Can you work these out from the drawing? Everything is in mm from the part's minimum corner. A direction names the side the tool comes from. Coordinates: 2 decimals unless noted, no trailing zeros. Order: outer loops, then holes, each group sorted by start corner. A loop starts at its lowest first (then second) coordinate and runs counter-clockwise, first axis right, second up. Notation, with made-up numbers: (9, 0.5) - (54, 0.5) arc R20 ccw to (54, 25.5) - close; hole circle Ø3 at (81, 55). An arc over 180 degrees is marked (long way). One line per item, written item: value.
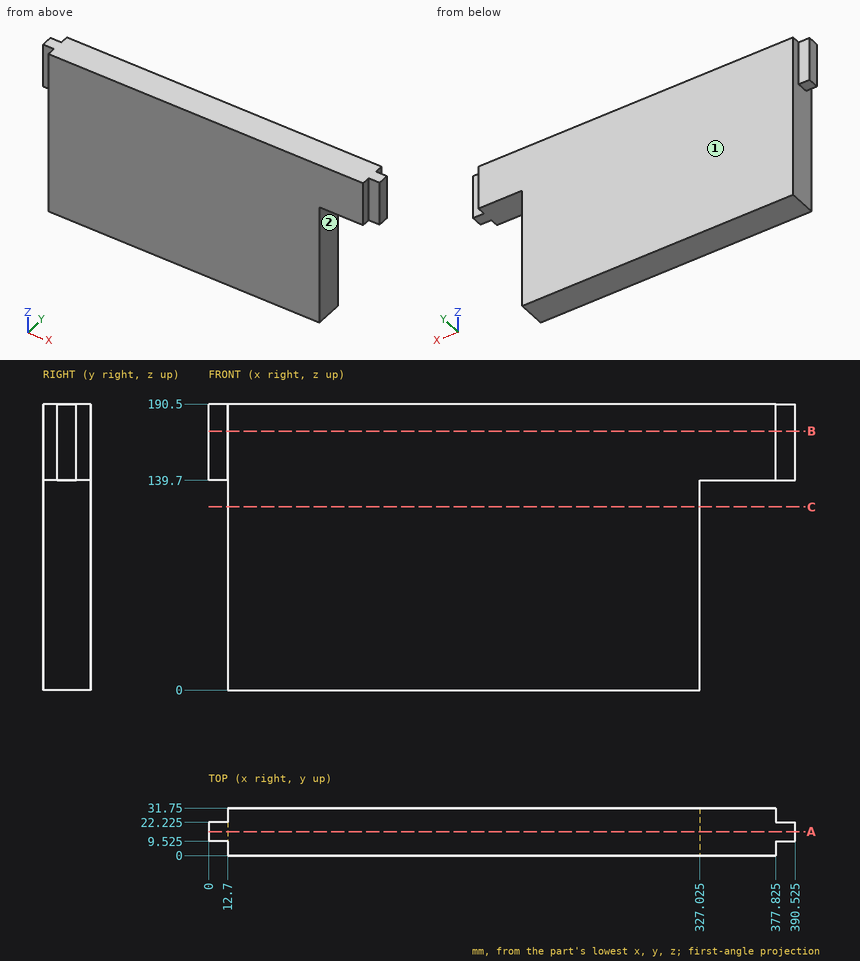
Item 1: I want a section at B-B on z = 172.5. Please give me the cut outline in (x, y) (3 decimals).
Conclusion:
outline: (0, 9.525) - (12.7, 9.525) - (12.7, 0) - (377.825, 0) - (377.825, 9.525) - (390.525, 9.525) - (390.525, 22.225) - (377.825, 22.225) - (377.825, 31.75) - (12.7, 31.75) - (12.7, 22.225) - (0, 22.225) - close
Item 2: I want a section at C-C on z = 122. Please give me the cut outline in (x, y) (3 decimals).
Conclusion:
outline: (12.7, 0) - (327.025, 0) - (327.025, 31.75) - (12.7, 31.75) - close
Item 3: I want a section at A-A on y = 16. Please give me the cut outline in (x, z) (3 decimals).
Conclusion:
outline: (0, 139.7) - (12.7, 139.7) - (12.7, 0) - (327.025, 0) - (327.025, 139.7) - (390.525, 139.7) - (390.525, 190.5) - (0, 190.5) - close
Item 4: For the marked faces 1 and 2, which set-ups out of +Z, -Z, +X, -X, +Y, -Y let a thin tool reach every point of the face, with its end or its side?
Conclusion:
face 1: +Z, -Z, +X, -X, +Y
face 2: -Z, +X, +Y, -Y
Item 5: I'm going to push flat-ended pins straight in: pin 1 Ø6.5 at (x, z) = (7.5, 177.5) entering from +Y (3 decimals); pin 2 Ø4 at (x, z) = (140, 48) entering from -Y; pin 3 Ø10.5 at (y, z) = (29, 160) entering from +X (3 decimals); pin 4 Ø9.5 at (y, z) = (14, 39.5) entering from +X (3 decimals). Where does each tip first touch, or does it pass through?
Conclusion:
pin 1: y = 22.225
pin 2: y = 0
pin 3: x = 377.825
pin 4: x = 327.025
Item 6: If I drill on probe 1 along X at (y, z) = (24, 176) (3 decimals); probe 2 along X at (y, z) = (3.5, 95) (3 decimals); probe 3 along Z at (x, y) = (371, 18.5), over which ranges is the centre line in solid material (lowest first)?
Conclusion:
probe 1: 12.7 to 377.825
probe 2: 12.7 to 327.025
probe 3: 139.7 to 190.5
